Work out the finished part from the listing and answer in its coordinate system (mm). A direction names the side the tool comes from. Give positions to 0.01 mm unless a question says otherwise; leave off trailing zeros. Loops run counter-clockwise (first coordinate to the right, second up) from the corner with the lowest first, then second, coordinate; pieces in that order, holes last. Notation, with made-up numbers: (-19, 25.25) - (-2, 25.25) arc R25 cw to (-2, 43.25) - close; hole circle Ø3 at (9, -40). An arc over 180 degrees is marked (long way). One line per question, with ' | ' between items. Start each with the question number.
1. Which of the six approach directions +Z, -Z, +X, -X, +Y, -Y give full straight-line access (tool end or side, diameter ignored) to faces 1 (the face through (0.13, -5.55, -8.74)), 2 (the face through (4, -12.7, -2))?
2. Find the intervals of material crossed by line 1 (Z direction, x = 0, y = -2.75) (3 decimals); line 2 (Z direction, x = 3, y = -5.5) (1 decimal); line 3 (X direction, y = -2.5, z = -2.25) (3 decimals), in increasing order.
3. For a pull along Y with two mould halves and no side action, classify faces 3 (the face through (9.525, -6, 0)), 4 (the face through (0.13, -7.13, -8.72)), 5 (the face through (-7.37, -0.25, -7.43)) as released by +Y, released by -Y, zero draft, split by the parting line, or undercut.
4. Section A-A (y = -2.25) is taken. Determine the outline of the cut face in (x, z) (1 decimal), plus the area to 3 significant figures.
from build123d import *

# Parameters (mm, degrees)
F0_R     = 3.96875
F1_DEPTH = 12.7
F3_DEPTH = 19.05


with BuildPart() as f1:
    # F0 (on Front) → F1 (new body)
    with BuildSketch(Plane.XZ):
        with BuildLine():
            Line((-9.525, 0), (-9.525, -9.525))
            Line((-9.525, -9.525), (0, -9.525))
            ThreePointArc((0, -9.525), (-6.7351920908, -6.7351920908), (-9.525, 0))
        make_face()
        with BuildLine():
            ThreePointArc((9.525, 0), (6.7351920908, -6.7351920908), (0, -9.525))
            Line((0, -9.525), (9.525, -9.525))
            Line((9.525, -9.525), (9.525, 0))
        make_face()
        with BuildLine():
            ThreePointArc((-9.525, 0), (-6.7351920908, -6.7351920908), (0, -9.525))
            ThreePointArc((0, -9.525), (6.7351920908, -6.7351920908), (9.525, 0))
            ThreePointArc((9.525, 0), (6.7351920908, 6.7351920908), (0, 9.525))
            ThreePointArc((0, 9.525), (-6.7351920908, 6.7351920908), (-9.525, 0))
        make_face()
        Circle(F0_R, mode=Mode.SUBTRACT)
        with BuildLine():
            Line((-9.525, 9.525), (-9.525, 0))
            ThreePointArc((-9.525, 0), (-6.7351920908, 6.7351920908), (0, 9.525))
            Line((0, 9.525), (-9.525, 9.525))
        make_face()
        with BuildLine():
            ThreePointArc((0, 9.525), (6.7351920908, 6.7351920908), (9.525, 0))
            Line((9.525, 0), (9.525, 9.525))
            Line((9.525, 9.525), (0, 9.525))
        make_face()
    extrude(amount=F1_DEPTH)

    # F2 (on face) → F3 (cut)
    with BuildSketch(Plane.YZ.offset(9.525)):
        Polygon((-4.7625, -9.525), (-6.35, -7.9375), (-7.9375, -9.525), align=None)
    extrude(amount=-F3_DEPTH, mode=Mode.SUBTRACT)

    # F5 (on mid) → F6 (revolve, cut)
    with BuildSketch(Plane.YZ):
        Polygon((-12.7, 20.5410033949), (-12.7, 9.525), (-9.7482707865, 20.5410033949), align=None)
        Polygon((-2.9517292135, 20.5410033949), (0, 9.525), (0, 20.5410033949), align=None)
    revolve(axis=Axis((0, 0, 0), (0, 1, 0)), mode=Mode.SUBTRACT)


solid = f1.part
Conclusion:
1) face 1: -Z, +X, -X | face 2: +Z, -Z, +X, -X, -Y
2) line 1: -9.525 to -3.969, 3.969 to 9.525 | line 2: -8.8 to -2.6, 2.6 to 9.5 | line 3: -9.525 to -3.269, 3.269 to 9.525
3) face 3: zero draft | face 4: undercut | face 5: released by +Y
4) outline: (-9.5, -9.5) - (9.5, -9.5) - (9.5, 9.5) - (-9.5, 9.5) - close; hole circle Ø7.9 at (0, 0) | area: 313 mm²
